from build123d import *

# Parameters (mm, degrees)
ESQUISSE1_R                  = 7
BOSS_EXTRU_1_DEPTH           = 160
ESQUISSE2_R                  = 4.188125
ENL_V_MAT_EXTRU_1_DEPTH      = 20
ENL_V_MAT_EXTRU_2_DEPTH      = 2.5
ENL_V_MAT_EXTRU_2_DEPTH_BACK = 2.5


with BuildPart() as part:
    # Esquisse1 → Boss.-Extru.1 (new body)
    with BuildSketch(Plane.XY):
        Circle(ESQUISSE1_R)
    extrude(amount=BOSS_EXTRU_1_DEPTH)

    # Esquisse2 → Enlèv. mat.-Extru.1 (cut)
    with BuildSketch(Plane(origin=(0, 0, 0), x_dir=(-1, 0, 0), z_dir=(0, 0, -1))):
        Circle(ESQUISSE2_R)
    extrude(amount=-ENL_V_MAT_EXTRU_1_DEPTH, mode=Mode.SUBTRACT)

    # Esquisse3 → Enlèv. mat.-Extru.2 (cut, two sides: drawn at the far end of the back side and taken through both)
    with BuildSketch(Plane.XZ.offset(-6.946049008).offset(-ENL_V_MAT_EXTRU_2_DEPTH_BACK)):
        with BuildLine():
            Line((2.5, 160), (2.5, 140))
            ThreePointArc((2.5, 140), (0, 137.5), (-2.5, 140))
            Line((-2.5, 140), (-2.5, 160))
            ThreePointArc((-2.5, 160), (0, 162.5), (2.5, 160))
        make_face()
    extrude(amount=ENL_V_MAT_EXTRU_2_DEPTH + ENL_V_MAT_EXTRU_2_DEPTH_BACK, mode=Mode.SUBTRACT)


solid = part.part
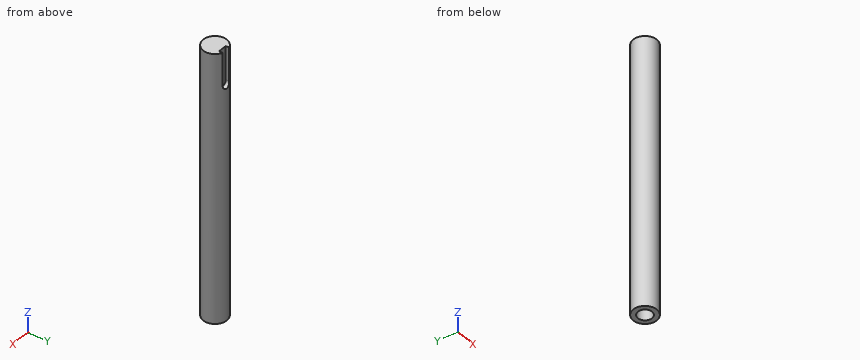
The listing builds one solid part. Answer for the finished solid, in the listing's coordinates (mm). Give positions to 0.01 mm unless a question says otherwise; leave off trailing zeros. Loops run counter-clockwise (first coordinate to the right, second up) from the corner with the lowest first, then second, coordinate; pieces in that order, holes last. Notation, with made-up numbers: (42, 47.5) - (71, 47.5) arc R22 ccw to (71, 70.5) - close; hole circle Ø8 at (51, 79). An arc over 180 degrees is marked (long way). Answer as a JSON object with one key per item and string values.
1. A cutting plane is placed at B-B (x = 0). Write down the section's boundary in (y, z).
Determined:
{"outline": "(-7, 0) - (-4.19, 0) - (-4.19, 20) - (4.19, 20) - (4.19, 0) - (7, 0) - (7, 137.5) - (4.45, 137.5) - (4.45, 160) - (-7, 160) - close"}
2. A cutting plane is placed at A-A (y = 0). Write down the section's boundary in (x, z), then the cut area to 3 significant figures.
Determined:
{"outline": "(-7, 0) - (-4.19, 0) - (-4.19, 20) - (4.19, 20) - (4.19, 0) - (7, 0) - (7, 160) - (-7, 160) - close", "area": "2,070 mm²"}
3. Flat-ended cylindrical pins translate along their axes: pin 1 Ø2.5 at (y, z) = (5.5, 152) entering from -X; pin 2 Ø3 at (y, z) = (-4, 112) entering from +X; pin 3 Ø2 at (y, z) = (-2.5, 42) entering from -X. Find the tip coordinate at first contact, or state that the pin passes through.
Determined:
{"pin 1": "x = -5.56", "pin 2": "x = 6.54", "pin 3": "x = -6.84"}
4. A cutting plane is placed at C-C (z = 118). Write down the section's boundary in (x, y).
Determined:
{"outline": "circle Ø14 at (0, 0)"}
5. Find the intervals of material crossed by L1, parallel to Y at x = 0, z = 4; L2, parallel to Z at x = 1.25, y = -3; L3, parallel to Y at x = -3.5, z = 29.5, in increasing order. Write a range as [from, to].
Determined:
{"L1": "[-7, -4.19], [4.19, 7]", "L2": "[20, 160]", "L3": "[-6.06, 6.06]"}
